from build123d import *

# Parameters (mm, degrees)
BASPROSKE_W              = 10
BASPROSKE_H              = 8.125
TOOTHCUT_DEPTH           = 16.232572009
TEETHCUTS_COUNT          = 11
TEETHCUTS_ANGLE          = 327.272727273
BORSKE_R                 = 3
BORE_DEPTH               = 50.0000508
RESSALTO_EXTRUS_O1_DEPTH = 10
RESSALTO_EXTRUS_O2_DEPTH = 5
ESBO_O3_R                = 1.35
CORTE_EXTRUS_O1_DEPTH    = 10


with BuildPart() as part:
    # BasProSke → Base-Revolve (revolve)
    with BuildSketch(Plane(origin=(0, 0, 0), x_dir=(1, 0, 0), z_dir=(0, 1, 0)), mode=Mode.PRIVATE) as base_revolve_sk:
        with Locations((5, 4.0625)):
            Rectangle(BASPROSKE_W, BASPROSKE_H)
    revolve(base_revolve_sk.sketch.rotate(Axis((-10, 0, 0), (1, 0, 0)), 180), axis=Axis((-10, 0, 0), (1, 0, 0)))

    # TooCutSke → ToothCut (cut, through all)
    with BuildSketch(Plane(origin=(0, 0, 0), x_dir=(0, 0, -1), z_dir=(1, 0, 0))):
        with BuildLine():
            ThreePointArc((0.716661614, 5.262929639), (0, 5.3115), (-0.716661614, 5.262929639))
            ThreePointArc((-0.716661614, 5.262929639), (-1.045232485, 6.771828733), (-2.135233901, 7.865735589))
            ThreePointArc((-2.135233901, 7.865735589), (0, 8.1504), (2.135233901, 7.865735589))
            ThreePointArc((2.135233901, 7.865735589), (1.045232485, 6.771828733), (0.716661614, 5.262929639))
        make_face()
    toothcut = extrude(amount=TOOTHCUT_DEPTH, mode=Mode.SUBTRACT)

    # TeethCuts: ToothCut ×11 about axis
    teethcuts_axis = Axis((-10, 0, 0), (1, 0, 0))
    for i in range(1, TEETHCUTS_COUNT):
        add(toothcut.rotate(teethcuts_axis, i * TEETHCUTS_ANGLE / (TEETHCUTS_COUNT - 1)), mode=Mode.SUBTRACT)

    # BorSke → Bore (cut, symmetric)
    with BuildSketch(Plane(origin=(0, 0, 0), x_dir=(0, 0, -1), z_dir=(1, 0, 0))):
        with Locations(Location((0, 0, 0), (0, 0, 180))):
            Circle(BORSKE_R)
    extrude(amount=BORE_DEPTH, both=True, mode=Mode.SUBTRACT)

    # Esboço1 → Ressalto-extrusão1 (add)
    with BuildSketch(Plane.ZY):
        with BuildLine():
            Line((-2.236067977, 2), (0, 2))
            Line((0, 2), (2.236067977, 2))
            ThreePointArc((2.236067977, 2), (0, 3), (-2.236067977, 2))
        make_face()
    extrude(amount=-RESSALTO_EXTRUS_O1_DEPTH)

    # Esboço2 → Ressalto-extrusão2 (add)
    with BuildSketch(Plane(origin=(10, 0, 0), x_dir=(0, 0, -1), z_dir=(1, 0, 0))):
        with BuildLine():
            ThreePointArc((5.499508602, -0.073519622), (5.499877149, -0.036760632), (5.5, 0))
            ThreePointArc((5.5, 0), (5.438664747, 0.819100589), (5.256026991, 1.619932181))
            ThreePointArc((5.256026991, 1.619932181), (5.169790583, 1.578653269), (5.085041182, 1.534401651))
            ThreePointArc((5.085041182, 1.534401651), (4.831510343, 2.206476842), (4.489617195, 2.838198318))
            ThreePointArc((4.489617195, 2.838198318), (4.578559391, 2.873268994), (4.666228749, 2.911410184))
            ThreePointArc((4.666228749, 2.911410184), (4.156622659, 3.601734037), (3.545849816, 4.204396399))
            ThreePointArc((3.545849816, 4.204396399), (3.495620198, 4.123047446), (3.448248696, 4.040001631))
            ThreePointArc((3.448248696, 4.040001631), (2.871613702, 4.46831814), (2.242460468, 4.814914672))
            ThreePointArc((2.242460468, 4.814914672), (2.298322765, 4.892503784), (2.351454238, 4.971987828))
            ThreePointArc((2.351454238, 4.971987828), (1.549529063, 5.277211355), (0.709890379, 5.453994467))
            ThreePointArc((0.709890379, 5.453994467), (0.711615099, 5.358403192), (0.716661614, 5.262929639))
            ThreePointArc((0.716661614, 5.262929639), (0, 5.3115), (-0.716661614, 5.262929639))
            ThreePointArc((-0.716661614, 5.262929639), (-0.711615099, 5.358403192), (-0.709890379, 5.453994467))
            ThreePointArc((-0.709890379, 5.453994467), (-1.549529063, 5.277211355), (-2.351454238, 4.971987828))
            ThreePointArc((-2.351454238, 4.971987828), (-2.298322765, 4.892503784), (-2.242460468, 4.814914672))
            ThreePointArc((-2.242460468, 4.814914672), (-2.871613702, 4.46831814), (-3.448248696, 4.040001631))
            ThreePointArc((-3.448248696, 4.040001631), (-3.495620198, 4.123047446), (-3.545849816, 4.204396399))
            ThreePointArc((-3.545849816, 4.204396399), (-4.156622659, 3.601734037), (-4.666228749, 2.911410184))
            ThreePointArc((-4.666228749, 2.911410184), (-4.578559391, 2.873268994), (-4.489617195, 2.838198318))
            ThreePointArc((-4.489617195, 2.838198318), (-4.831510343, 2.206476842), (-5.085041182, 1.534401651))
            ThreePointArc((-5.085041182, 1.534401651), (-5.169790583, 1.578653269), (-5.256026991, 1.619932181))
            ThreePointArc((-5.256026991, 1.619932181), (-5.44401793, 0.782731611), (-5.499508602, -0.073519622))
            ThreePointArc((-5.499508602, -0.073519622), (-5.405135761, -0.0582084), (-5.311352185, -0.039625949))
            ThreePointArc((-5.311352185, -0.039625949), (-5.257436589, -0.755905263), (-5.107369022, -1.458360012))
            ThreePointArc((-5.107369022, -1.458360012), (-5.202588986, -1.466952167), (-5.297452733, -1.478849059))
            ThreePointArc((-5.297452733, -1.478849059), (-5.002975974, -2.284782572), (-4.586733332, -3.035107468))
            ThreePointArc((-4.586733332, -3.035107468), (-4.515619718, -2.971205038), (-4.446770385, -2.904869256))
            ThreePointArc((-4.446770385, -2.904869256), (-4.014163864, -3.478292788), (-3.508143284, -3.988102675))
            ThreePointArc((-3.508143284, -3.988102675), (-3.583602145, -4.046810655), (-3.656974663, -4.108106171))
            ThreePointArc((-3.656974663, -4.108106171), (-2.973524496, -4.626894431), (-2.217702637, -5.033070138))
            ThreePointArc((-2.217702637, -5.033070138), (-2.19242632, -4.940865071), (-2.170370406, -4.8478371))
            ThreePointArc((-2.170370406, -4.8478371), (-1.496422476, -5.096346929), (-0.795106841, -5.251650918))
            ThreePointArc((-0.795106841, -5.251650918), (-0.826846944, -5.341835354), (-0.855432976, -5.433068601))
            ThreePointArc((-0.855432976, -5.433068601), (0, -5.5), (0.855432976, -5.433068601))
            ThreePointArc((0.855432976, -5.433068601), (0.826846944, -5.341835354), (0.795106841, -5.251650918))
            ThreePointArc((0.795106841, -5.251650918), (1.496422476, -5.096346929), (2.170370406, -4.8478371))
            ThreePointArc((2.170370406, -4.8478371), (2.19242632, -4.940865071), (2.217702637, -5.033070138))
            ThreePointArc((2.217702637, -5.033070138), (2.973524496, -4.626894431), (3.656974663, -4.108106171))
            ThreePointArc((3.656974663, -4.108106171), (3.583602145, -4.046810655), (3.508143284, -3.988102675))
            ThreePointArc((3.508143284, -3.988102675), (4.014163864, -3.478292788), (4.446770385, -2.904869256))
            ThreePointArc((4.446770385, -2.904869256), (4.515619718, -2.971205038), (4.586733332, -3.035107468))
            ThreePointArc((4.586733332, -3.035107468), (5.002975974, -2.284782572), (5.297452733, -1.478849059))
            ThreePointArc((5.297452733, -1.478849059), (5.202588986, -1.466952167), (5.107369022, -1.458360012))
            ThreePointArc((5.107369022, -1.458360012), (5.257436589, -0.755905263), (5.311352185, -0.039625949))
            ThreePointArc((5.311352185, -0.039625949), (5.405135761, -0.0582084), (5.499508602, -0.073519622))
        make_face()
        with BuildLine():
            Line((-2.236067977, 2), (2.236067977, 2))
            ThreePointArc((2.236067977, 2), (0, -3), (-2.236067977, 2))
        make_face(mode=Mode.SUBTRACT)
        with BuildLine():
            ThreePointArc((3.448248696, 4.040001631), (3.495620198, 4.123047446), (3.545849816, 4.204396399))
            ThreePointArc((3.545849816, 4.204396399), (2.973524496, 4.626894431), (2.351454238, 4.971987828))
            ThreePointArc((2.351454238, 4.971987828), (2.298322765, 4.892503784), (2.242460468, 4.814914672))
            ThreePointArc((2.242460468, 4.814914672), (2.871613702, 4.46831814), (3.448248696, 4.040001631))
        make_face()
        with BuildLine():
            ThreePointArc((0.716661614, 5.262929639), (0.711615099, 5.358403192), (0.709890379, 5.453994467))
            ThreePointArc((0.709890379, 5.453994467), (0, 5.5), (-0.709890379, 5.453994467))
            ThreePointArc((-0.709890379, 5.453994467), (-0.711615099, 5.358403192), (-0.716661614, 5.262929639))
            ThreePointArc((-0.716661614, 5.262929639), (0, 5.3115), (0.716661614, 5.262929639))
        make_face()
        with BuildLine():
            ThreePointArc((-2.242460468, 4.814914672), (-2.298322765, 4.892503784), (-2.351454238, 4.971987828))
            ThreePointArc((-2.351454238, 4.971987828), (-2.973524496, 4.626894431), (-3.545849816, 4.204396399))
            ThreePointArc((-3.545849816, 4.204396399), (-3.495620198, 4.123047446), (-3.448248696, 4.040001631))
            ThreePointArc((-3.448248696, 4.040001631), (-2.871613702, 4.46831814), (-2.242460468, 4.814914672))
        make_face()
        with BuildLine():
            ThreePointArc((-4.489617195, 2.838198318), (-4.578559391, 2.873268994), (-4.666228749, 2.911410184))
            ThreePointArc((-4.666228749, 2.911410184), (-5.002975974, 2.284782572), (-5.256026991, 1.619932181))
            ThreePointArc((-5.256026991, 1.619932181), (-5.169790583, 1.578653269), (-5.085041182, 1.534401651))
            ThreePointArc((-5.085041182, 1.534401651), (-4.831510343, 2.206476842), (-4.489617195, 2.838198318))
        make_face()
        with BuildLine():
            ThreePointArc((-5.311352185, -0.039625949), (-5.405135761, -0.0582084), (-5.499508602, -0.073519622))
            ThreePointArc((-5.499508602, -0.073519622), (-5.44401793, -0.782731611), (-5.297452733, -1.478849059))
            ThreePointArc((-5.297452733, -1.478849059), (-5.202588986, -1.466952167), (-5.107369022, -1.458360012))
            ThreePointArc((-5.107369022, -1.458360012), (-5.257436589, -0.755905263), (-5.311352185, -0.039625949))
        make_face()
        with BuildLine():
            ThreePointArc((-4.586733332, -3.035107468), (-4.156622659, -3.601734037), (-3.656974663, -4.108106171))
            ThreePointArc((-3.656974663, -4.108106171), (-3.583602145, -4.046810655), (-3.508143284, -3.988102675))
            ThreePointArc((-3.508143284, -3.988102675), (-4.014163864, -3.478292788), (-4.446770385, -2.904869256))
            ThreePointArc((-4.446770385, -2.904869256), (-4.515619718, -2.971205038), (-4.586733332, -3.035107468))
        make_face()
        with BuildLine():
            ThreePointArc((-2.217702637, -5.033070138), (-1.549529063, -5.277211355), (-0.855432976, -5.433068601))
            ThreePointArc((-0.855432976, -5.433068601), (-0.826846944, -5.341835354), (-0.795106841, -5.251650918))
            ThreePointArc((-0.795106841, -5.251650918), (-1.496422476, -5.096346929), (-2.170370406, -4.8478371))
            ThreePointArc((-2.170370406, -4.8478371), (-2.19242632, -4.940865071), (-2.217702637, -5.033070138))
        make_face()
        with BuildLine():
            ThreePointArc((0.855432976, -5.433068601), (1.549529063, -5.277211355), (2.217702637, -5.033070138))
            ThreePointArc((2.217702637, -5.033070138), (2.19242632, -4.940865071), (2.170370406, -4.8478371))
            ThreePointArc((2.170370406, -4.8478371), (1.496422476, -5.096346929), (0.795106841, -5.251650918))
            ThreePointArc((0.795106841, -5.251650918), (0.826846944, -5.341835354), (0.855432976, -5.433068601))
        make_face()
        with BuildLine():
            ThreePointArc((3.656974663, -4.108106171), (4.156622659, -3.601734037), (4.586733332, -3.035107468))
            ThreePointArc((4.586733332, -3.035107468), (4.515619718, -2.971205038), (4.446770385, -2.904869256))
            ThreePointArc((4.446770385, -2.904869256), (4.014163864, -3.478292788), (3.508143284, -3.988102675))
            ThreePointArc((3.508143284, -3.988102675), (3.583602145, -4.046810655), (3.656974663, -4.108106171))
        make_face()
        with BuildLine():
            ThreePointArc((5.297452733, -1.478849059), (5.44401793, -0.782731611), (5.499508602, -0.073519622))
            ThreePointArc((5.499508602, -0.073519622), (5.405135761, -0.0582084), (5.311352185, -0.039625949))
            ThreePointArc((5.311352185, -0.039625949), (5.257436589, -0.755905263), (5.107369022, -1.458360012))
            ThreePointArc((5.107369022, -1.458360012), (5.202588986, -1.466952167), (5.297452733, -1.478849059))
        make_face()
        with BuildLine():
            ThreePointArc((5.085041182, 1.534401651), (5.169790583, 1.578653269), (5.256026991, 1.619932181))
            ThreePointArc((5.256026991, 1.619932181), (5.002975974, 2.284782572), (4.666228749, 2.911410184))
            ThreePointArc((4.666228749, 2.911410184), (4.578559391, 2.873268994), (4.489617195, 2.838198318))
            ThreePointArc((4.489617195, 2.838198318), (4.831510343, 2.206476842), (5.085041182, 1.534401651))
        make_face()
    extrude(amount=RESSALTO_EXTRUS_O2_DEPTH)

    # Esboço3 → Corte-extrusão1 (cut)
    with BuildSketch(Plane.XZ.offset(-2)):
        with Locations(Location((11.990687454, 0, 0), (0, 0, 270))):
            Circle(ESBO_O3_R)
    extrude(amount=-CORTE_EXTRUS_O1_DEPTH, mode=Mode.SUBTRACT)


solid = part.part
Geometry: final body of the model. Coordinates: model frame, mm. A direction names the side the tool comes from. Round coordinates to 2 decimals unless told otherwise and drop trailing zeros. Loops run counter-clockwise (first coordinate to the right, second up) from the corner with the lowest first, then second, coordinate; pieces in that order, holes last.
Q1. Section C-C on z = -5.75. Return loops of the section in (x, y).
Q2. Material intervals for L1, parallel to Y at x = 1.25, z = 0 (1 decimal); L2, parallel to Z at x = 1.25, y = -6.5; L3, parallel to X at y = 4.7, z = 0, sorted ascending.
Q3. Section B-B on y = -1.75. Return loops of the section in (x, z).
Q4. Section D-D on y = -5.75. Return loops of the section in (x, z), plus the area to 3 significant figures.
Q5. Access query for faces 3 (the flat face through (10, -3, 6)), 4 (the flat face through (10, -6, -4)). Directions: +Z, -Z, +X, -X, +Y, -Y. A direction counts if a zero-diameter tool reaches every point of the face in a straight line with its end or side. Return the directions, or none.
Q6. Pin query (flat end, axial travel): P1, Ø0.6, axis at y = 7, z = 1.5, coming from the +X side; P2, Ø5, axis at x = 11.5, y = 4.5, coming from the -Z side (3 decimals); P3, Ø4, axis at x = 9, y = 5, coming from the +Z side (3 decimals). Return the tip coordinate at first contact, or that it passes through.
Q7. Pull-direction query (Y, two-part tool) for faces 1 (the cylindrical face through (4.93, -6.753, 0.913)), 2 (the cylindrical face through (10.673, 3.726, 0.293)); classes: released by +Y, released by -Y, zero draft, split by the parting line, or undercut.
Q8. Section A-A on y = 4.5. Return loops of the section in (x, z), plus the area to 3 significant figures.
Evaluation:
1. outline: (0, -3.63) - (10, -3.63) - (10, -1.58) - (0, -1.58) - close; (0, -0.1) - (10, -0.1) - (10, 1.79) - (0, 1.79) - close; (0, 3.8) - (10, 3.8) - (10, 5.47) - (0, 5.47) - close
2. L1: y = -8.1 to -3, 2 to 5.3
2. L2: z = -4.59 to -3.26, -0.95 to 0.95, 3.26 to 4.59
2. L3: x = 0 to 10.64, 13.34 to 15
3. outline: (0, -6.15) - (10, -6.15) - (10, -5.21) - (15, -5.21) - (15, -2.44) - (0, -2.44) - close; (0, 2.44) - (15, 2.44) - (15, 5.21) - (10, 5.21) - (10, 6.15) - (0, 6.15) - close
4. outline: (0, -4.57) - (10, -4.57) - (10, -2.55) - (0, -2.55) - close; (0, -0.93) - (10, -0.93) - (10, 0.93) - (0, 0.93) - close; (0, 2.55) - (10, 2.55) - (10, 4.57) - (0, 4.57) - close
4. area: 59.1 mm2
5. face 3: +Z, +X, -Y
5. face 4: -Z, +X, -Y
6. P1: stops at x = 10
6. P2: stops at z = -6.265
6. P3: stops at z = 6.265
7. face 1: undercut
7. face 2: zero draft
8. outline: (0, -6.12) - (10, -6.12) - (10, -3.76) - (0, -3.76) - close; (0, -2.82) - (10, -2.82) - (10, -3.16) - (15, -3.16) - (15, 3.16) - (10, 3.16) - (10, 2.82) - (0, 2.82) - close; (0, 3.76) - (10, 3.76) - (10, 6.12) - (0, 6.12) - close; hole circle Ø2.7 at (11.99, 0)
8. area: 129 mm2
